Autodesk Inventor part; units mm, degrees
ref_plane "YZ Plane" through (0, 0, 0) normal (1, 0, 0) x (0, 1, 0)
ref_plane "XZ Plane" through (0, 0, 0) normal (0, 1, 0) x (-1, 0, 0)
ref_plane "XY Plane" through (0, 0, 0) normal (0, 0, 1) x (1, 0, 0)
sketch "Sketch1" plane through (0, 0, 0) normal (0, 1, 0) x (-1, 0, 0)
  line L0 (0, 0) -> (138, 0)
  line L1 (138, 0) -> (138, -67)
  line L2 (138, -67) -> (0, -67)
  line L3 (0, -67) -> (0, 0)
  dimension "d0" = 138
  dimension "d1" = 67
extrude "Extrusion1" add sketch "Sketch1" along normal blind 8
fillet "Fillet3" radius 9 4 edges at (-138, 4, 0) (-138, 4, -67) (0, 4, 0) (0, 4, -67)
fillet "Fillet4" radius 2.5 16 edges at (-135.364, 8, -2.636) (-69, 8, 0) (-2.636, 8, -2.636) (0, 8, -33.5) (-2.636, 8, -64.364) (-69, 8, -67) (-135.364, 8, -64.364) (-138, 8, -33.5) (0, 0, -33.5) (-2.636, 0, -64.364) (-69, 0, -67) (-135.364, 0, -64.364) (-138, 0, -33.5) (-135.364, 0, -2.636) (-69, 0, 0) (-2.636, 0, -2.636)
sketch "Sketch9" plane through (0, 8, 0) normal (0, 1, 0) x (1, 0, 0)
  line L0 (-135.5, 9) -> (-135.5, 58)
  line L1 (-2.5, 58) -> (-2.5, 9)
  line L2 (-9, 2.5) -> (-129, 2.5)
  line L3 (-129, 64.5) -> (-9, 64.5)
  line L4 (-121, 4.5) -> (-17, 4.5)
  line L5 (-17, 4.5) -> (-17, 62.5)
  line L6 (-17, 62.5) -> (-121, 62.5)
  line L7 (-121, 62.5) -> (-121, 4.5)
  point P0 (0, 0)
sketch "Sketch11" plane through (0, 8, 0) normal (0, 1, 0) x (1, 0, 0)
  line L0 (-2.5, 58) -> (-2.5, 9)
  circle A0 centre (-9.7532, 33.5) radius 4.75
  line L1 (-135.5, 9) -> (-135.5, 58)
  circle A1 centre (-133.0353, 33.5) radius 0.5
  line L2 (-129.849, 33.5) -> (-129.849, 38)
  line L3 (-129.849, 38) -> (-130.449, 38)
  line L4 (-130.449, 38) -> (-130.449, 33.5)
  line L5 (-130.449, 33.5) -> (-130.449, 29)
  line L6 (-130.449, 29) -> (-129.849, 29)
  line L7 (-129.849, 29) -> (-129.849, 33.5)
  circle A2 centre (-130.149, 27.1522) radius 0.5173
  line L8 (-130.449, 29) -> (-129.849, 29)
  line L9 (-129.849, 29) -> (-129.849, 38)
  line L10 (-129.849, 38) -> (-130.449, 38)
  line L11 (-130.449, 38) -> (-130.449, 29)
  point P0 (0, 0)
  dimension "d21" = 9.5
  dimension "d22" = 1
extrude "Extrusion2" cut sketch "Sketch11" against normal blind 0.3
sketch "Sketch12" plane through (0, 8, 0) normal (0, 1, 0) x (1, 0, 0)
  line L0 (-121.0067, 4.7801) -> (-121.0067, 62.5653) construction
  line L1 (-121.0067, 62.5653) -> (-18.2774, 62.5653) construction
  line L2 (-18.2774, 62.5653) -> (-18.2774, 4.7801) construction
  line L3 (-18.2774, 4.7801) -> (-121.0067, 4.7801) construction
  point P0 (0, 0)
sketch "Sketch15" plane through (0, 2.5, -58) normal (1, 0, 0) x (0, 0, -1)
  line L0 (-49, 0) -> (-49, 3)
  line L1 (0, 3) -> (0, 0)
  circle A0 centre (-3.6879, 1.5) radius 0.7
  circle A1 centre (-5.8468, 1.5) radius 0.7
  circle A2 centre (-8.0674, 1.5) radius 0.7
  circle A3 centre (-10.3497, 1.5) radius 0.7
  circle A4 centre (-12.5703, 1.5) radius 0.7
  point P0 (-58, -2.5)
extrude "Extrusion5" cut sketch "Sketch15" against normal blind 0.6
sketch "Sketch16" plane through (0, 2.5, -58) normal (1, 0, 0) x (0, 0, -1)
  point P0 (-58, -2.5)
sketch "Sketch17" plane through (0, 2.5, -58) normal (1, 0, 0) x (0, 0, -1)
  line L0 (-49, 0) -> (-49, 3)
  line L1 (-49, 1.5) -> (0, 1.5)
  line L2 (0, 3) -> (0, 0)
  line L3 (-49, 3) -> (0, 3)
  line L4 (-24.5, 3) -> (-24.5, 0)
  circle A0 centre (-46.1363, 1.5) radius 1.15
  line L5 (-27.6835, 2.2868) -> (-21.9014, 2.2868)
  line L6 (-21.2014, 1.5868) -> (-21.2014, 1.4809)
  line L7 (-21.9014, 0.7809) -> (-27.6835, 0.7809)
  line L8 (-28.3835, 1.4809) -> (-28.3835, 1.5868)
  arc A1 (-27.6835, 2.2868) -> (-28.3835, 1.5868) centre (-27.6835, 1.5868) ccw
  arc A2 (-28.3835, 1.4809) -> (-27.6835, 0.7809) centre (-27.6835, 1.4809) ccw
  arc A3 (-21.2014, 1.5868) -> (-21.9014, 2.2868) centre (-21.9014, 1.5868) ccw
  arc A4 (-21.9014, 0.7809) -> (-21.2014, 1.4809) centre (-21.9014, 1.4809) ccw
  point P0 (-58, -2.5)
  dimension "d67" = 0.7
  dimension "d68" = 0.7
extrude "Extrusion6" cut sketch "Sketch17" against normal blind 4 contours A0 L1 | L1 A0 | L5 A3 L6 L1 L4 | L4 L1 L8 A1 L5 | L1 L4 L7 A2 L8 | L1 L6 A4 L7 L4
sketch "Sketch18" plane through (-129, 2.5, 0) normal (0, 0, 1) x (1, 0, 0)
  line L0 (0, 0) -> (0, 3)
  line L1 (0, 1.5) -> (120, 1.5)
  line L2 (120, 0) -> (129, 0)
  line L3 (17.633, 1.989) -> (25.3803, 1.989)
  line L4 (25.8803, 1.489) -> (25.8803, 1.2394)
  line L5 (25.3803, 0.7394) -> (17.633, 0.7394)
  line L6 (17.133, 1.2394) -> (17.133, 1.489)
  line L7 (29.1572, 1.989) -> (36.4879, 1.989)
  line L8 (36.9879, 1.489) -> (36.9879, 1.2394)
  line L9 (36.4879, 0.7394) -> (29.1572, 0.7394)
  line L10 (28.6572, 1.2394) -> (28.6572, 1.489)
  arc A0 (17.633, 1.989) -> (17.133, 1.489) centre (17.633, 1.489) ccw
  arc A1 (17.133, 1.2394) -> (17.633, 0.7394) centre (17.633, 1.2394) ccw
  arc A2 (25.8803, 1.489) -> (25.3803, 1.989) centre (25.3803, 1.489) ccw
  arc A3 (25.3803, 0.7394) -> (25.8803, 1.2394) centre (25.3803, 1.2394) ccw
  arc A4 (29.1572, 1.989) -> (28.6572, 1.489) centre (29.1572, 1.489) ccw
  arc A5 (28.6572, 1.2394) -> (29.1572, 0.7394) centre (29.1572, 1.2394) ccw
  arc A6 (36.9879, 1.489) -> (36.4879, 1.989) centre (36.4879, 1.489) ccw
  arc A7 (36.4879, 0.7394) -> (36.9879, 1.2394) centre (36.4879, 1.2394) ccw
  point P0 (129, -2.5)
  point P1 (28.6572, 1.989)
  point P2 (36.9879, 0.7394)
  dimension "d71" = 0.5
extrude "Extrusion7" add sketch "Sketch18" along normal blind 0.5
sketch "Sketch19" plane through (-129, 2.5, 0) normal (0, 0, 1) x (1, 0, 0)
  line L0 (12.7221, 0.7394) -> (8.2034, 0.7394)
  line L1 (7.9034, 1.0394) -> (7.9034, 1.6002)
  line L2 (8.2034, 1.9002) -> (12.7221, 1.9002)
  line L3 (13.0221, 1.6002) -> (13.0221, 1.0394)
  arc A0 (8.2034, 1.9002) -> (7.9034, 1.6002) centre (8.2034, 1.6002) ccw
  arc A1 (7.9034, 1.0394) -> (8.2034, 0.7394) centre (8.2034, 1.0394) ccw
  arc A2 (13.0221, 1.6002) -> (12.7221, 1.9002) centre (12.7221, 1.6002) ccw
  arc A3 (12.7221, 0.7394) -> (13.0221, 1.0394) centre (12.7221, 1.0394) ccw
  point P0 (129, -2.5)
  dimension "d74" = 0.3
extrude "Extrusion8" cut sketch "Sketch19" against normal blind 0.7
sketch "Sketch20" plane through (-129, 2.5, -0.7) normal (0, 0, 1) x (1, 0, 0)
  line L0 (12.7071, 1.7577) -> (8.1711, 1.7577)
  line L1 (8.0711, 1.6577) -> (8.0711, 1.5231)
  line L2 (8.1711, 1.4231) -> (12.7071, 1.4231)
  line L3 (12.8071, 1.5231) -> (12.8071, 1.6577)
  arc A0 (12.8071, 1.6577) -> (12.7071, 1.7577) centre (12.7071, 1.6577) ccw
  arc A1 (12.7071, 1.4231) -> (12.8071, 1.5231) centre (12.7071, 1.5231) ccw
  arc A2 (8.1711, 1.7577) -> (8.0711, 1.6577) centre (8.1711, 1.6577) ccw
  arc A3 (8.0711, 1.5231) -> (8.1711, 1.4231) centre (8.1711, 1.5231) ccw
  point P0 (129, -2.5)
  dimension "d77" = 0.1
  dimension "d78" = 0.1
extrude "Extrusion9" add sketch "Sketch20" along normal blind 0.9
sketch "Sketch21" plane through (-9, 2.5, -67) normal (0, 0, -1) x (-1, 0, 0)
  line L0 (107.2779, 0.7394) -> (111.7966, 0.7394)
  line L1 (102.367, 1.989) -> (94.6197, 1.989)
  line L2 (109.0372, 0.7394) -> (102.3642, 0.7394)
  line L3 (101.8642, 1.2394) -> (101.8642, 1.489)
  line L4 (102.3642, 1.989) -> (109.0372, 1.989)
  line L5 (109.5372, 1.489) -> (109.5372, 1.2394)
  arc A0 (101.8642, 1.2394) -> (102.3642, 0.7394) centre (102.3642, 1.2394) ccw
  arc A1 (102.3642, 1.989) -> (101.8642, 1.489) centre (102.3642, 1.489) ccw
  arc A2 (109.0372, 0.7394) -> (109.5372, 1.2394) centre (109.0372, 1.2394) ccw
  arc A3 (109.5372, 1.489) -> (109.0372, 1.989) centre (109.0372, 1.489) ccw
  point P0 (-9, -2.5)
  point P1 (109.5372, 0.7394)
  point P2 (101.8642, 1.989)
  dimension "d81" = 0.5
extrude "Extrusion10" add sketch "Sketch21" along normal blind 0.5
sketch "Sketch22" plane through (0, 0, 0) normal (0, -1, 0) x (1, 0, 0)
  point P0 (0, 0)
sketch "Sketch23" plane through (0, 0, 0) normal (0, -1, 0) x (1, 0, 0)
  circle A0 centre (-128.9815, -54.6956) radius 3.03
  circle A1 centre (-128.9815, -48.6898) radius 1.1168
  point P0 (0, 0)
extrude "Extrusion11" add sketch "Sketch23" along normal blind 1 contours A0
sketch "Sketch24" plane through (-128.9815, -1, -54.6956) normal (0, -1, 0) x (1, 0, 0)
  circle A0 centre (0, 0) radius 2.5382
  point P0 (128.9815, 54.6956)
extrude "Extrusion12" cut sketch "Sketch24" against normal blind 0.3
sketch "Sketch25" plane through (-128.9815, -0.7, -54.6956) normal (0, -1, 0) x (1, 0, 0)
  circle A0 centre (0, 0) radius 1.6518
  point P0 (128.9815, 54.6956)
extrude "Extrusion13" add sketch "Sketch25" along normal blind 0.3
sketch "Sketch26" plane through (-128.9815, -1, -54.6956) normal (0, -1, 0) x (1, 0, 0)
  circle A0 centre (0, 0) radius 0.4872
  point P0 (128.9815, 54.6956)
extrude "Extrusion14" cut sketch "Sketch26" against normal blind 0.3
sketch "Sketch27" plane through (0, 0, 0) normal (0, -1, 0) x (1, 0, 0)
  circle A0 centre (-128.9815, -49.2163) radius 0.9142
  point P0 (0, 0)
extrude "Extrusion15" cut sketch "Sketch27" against normal blind 0.3
sketch "Sketch28" plane through (0, 0, 0) normal (0, -1, 0) x (1, 0, 0)
  line L0 (-105.2991, -46.5746) -> (-105.2991, -22.5188) construction
  line L1 (-105.2991, -22.5188) -> (-81.2433, -22.5188) construction
  line L2 (-81.2433, -22.5188) -> (-81.2433, -46.5746) construction
  line L3 (-81.2433, -46.5746) -> (-105.2991, -46.5746) construction
  point P0 (0, 0)
properties part number "telefon"
Geometry check sheet. Reference: the model listing, model coordinates, mm. A direction names the side the tool comes from. Coordinates: 2 decimals unless noted, no trailing zeros. Order: outer loops, then holes, each group sorted by start corner. A loop starts at its lowest first (then second) coordinate and runs counter-clockwise, first axis right, second up. Notation, with made-up numbers: (36, 39) - (93, 39) arc R33 cw to (93, 76) - close; hole circle Ø10 at (-36, -6.5). An arc over 180 degrees is marked (long way). One line per item, written item: value.
(1) Sectioned sample at A-A (x = -55). Enter the section's corners in (y, z).
Data:
outline: (0, -64.5) arc R2.5 ccw to (2.5, -67) - (5.5, -67) arc R2.5 ccw to (8, -64.5) - (8, -2.5) arc R2.5 ccw to (5.5, 0) - (2.5, 0) arc R2.5 ccw to (0, -2.5) - close
(2) Depth check by flat-ended pin: pin 1 Ø0.6 at (x, z) = (-118.5, -0.5) entering from -Y; pin 2 Ø8 at (x, z) = (-53, -22) entering from -Y; pin 3 Ø3 at (y, z) = (1.5, -36.5) entering from -X; pin 4 Ø0.6 at (x, z) = (-109, 0) entering from +Y. Enter the tip coordinate at first touch or a pass-through.
Data:
pin 1: stops at y = 0.67
pin 2: stops at y = 0
pin 3: stops at x = -138
pin 4: stops at y = 6.69
(3) Access from +Z, -Z, +X, -X, +Y, -Y to the whole of each face (thin tool, end or side, straight path). Record for faces 4 (the face through (-135.294, 4.021, -64.434)), 5 (the face through (-68, 8, -33)), 6 (the face through (-132.01, -0.49, -54.83)), 7 (the face through (-2, 3.281, -33)), 8 (the face through (-10, 7.7, -34)).
Data:
face 4: -Z, -X, +Y, -Y
face 5: +Z, -Z, +X, -X, +Y
face 6: -Y
face 7: +X
face 8: +Y
(4) Release check for a two-part mould opening along X. For faces 1 (the face through (-68.16, 7.248, -66.287)), 2 (the face through (0, 3, -34)), 3 (the face through (-126.56, -0.85, -53.93)) record: +X half, -X half, draft (parallel to the pull), parting line (faces both ways), or undercut.
Data:
face 1: draft
face 2: +X half
face 3: undercut
(5) Thickness scan on probe 1 along Z at (x, y) = (-2.4, 4); probe 2 along Y at (x, z) = (-74, -29); probe 3 along X at (y, z) = (4, -11). Record the ranges inside material, lowest first. Write a range as from..to.
Data:
probe 1: z = -64.12..-36.8, -29.62..-13.01, -10.71..-2.88
probe 2: y = 0..8
probe 3: x = -138..-4
